For this review, take the finished solid that the model builds, in its own axes (mm). Give positions to 0.01 mm unless a question says otherwise; leave off trailing zeros. Loops run counter-clockwise (first coordinate to the right, second up) from the corner with the lowest first, then second, coordinate; pieces in that order, holes last. Notation, with made-up numbers: (41.5, 16) - (77.5, 16) arc R24 cw to (77.5, 30) - close; hole circle Ø2 at (77, -2). An arc over 180 degrees is marked (long way). Answer in a Markdown table with one row per item.
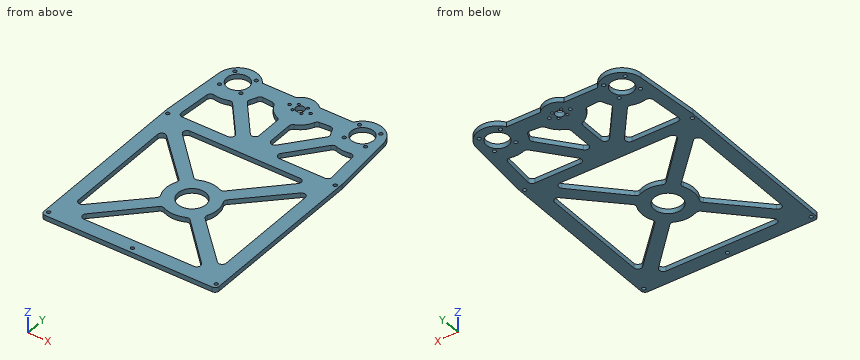
```python
from build123d import *

# Parameters (mm, degrees)
F0_R     = 2.25
F0_R_2   = 17.5
F0_R_3   = 14
F0_R_4   = 1.75
F0_R_5   = 2
F0_R_6   = 5.475
F1_DEPTH = 6


with BuildPart() as f1:
    # F0 (on Top) → F1 (new body)
    with BuildSketch(Plane.XY):
        with BuildLine():
            ThreePointArc((-94.039087, -168.43725), (-92.574621, -171.972784), (-89.039087, -173.43725))
            Line((-89.039087, -173.43725), (120.995737, -173.43725))
            ThreePointArc((120.995737, -173.43725), (124.531271, -171.972784), (125.995737, -168.43725))
            Line((125.995737, -168.43725), (125.995737, 46.355272))
            ThreePointArc((125.995737, 46.355272), (125.98705, 46.77201), (125.961003, 47.188025))
            Line((125.961003, 47.188025), (119.17908, 128.344968))
            ThreePointArc((119.17908, 128.344968), (119.244197, 127.304932), (119.265916, 126.263086))
            ThreePointArc((119.265916, 126.263086), (94.265916, 101.263086), (69.265916, 126.263086))
            ThreePointArc((69.265916, 126.263086), (70.26509, 133.260256), (73.182747, 139.698115))
            Line((73.182747, 139.698115), (30.811448, 139.698115))
            ThreePointArc((30.811448, 139.698115), (15.995916, 146.263086), (1.180383, 139.698115))
            Line((1.180383, 139.698115), (-41.190916, 139.698115))
            ThreePointArc((-41.190916, 139.698115), (-68.259772, 150.535942), (-87.186355, 128.355636))
            Line((-87.186355, 128.355636), (-94.003995, 47.190147))
            ThreePointArc((-94.003995, 47.190147), (-94.03031, 46.772005), (-94.039087, 46.353127))
            Line((-94.039087, 46.353127), (-94.039087, -168.43725))
        make_face()
        with Locations((-89.234084, -166.810914)):
            Circle(F0_R, mode=Mode.SUBTRACT)
        with BuildLine():
            ThreePointArc((-76.734085, 6.31898), (-73.661072, 10.932734), (-68.219396, 9.875237))
            Line((-68.219396, 9.875237), (-14.42265, -43.292696))
            ThreePointArc((-14.42265, -43.292696), (-13.014402, -45.974488), (-13.412905, -48.977214))
            ThreePointArc((-13.412905, -48.977214), (-16.504084, -62.810914), (-13.412905, -76.644614))
            ThreePointArc((-13.412905, -76.644614), (-13.014402, -79.64734), (-14.42265, -82.329132))
            Line((-14.42265, -82.329132), (-68.219396, -135.497065))
            ThreePointArc((-68.219396, -135.497065), (-73.661072, -136.554562), (-76.734085, -131.940809))
            Line((-76.734085, -131.940809), (-76.734085, 6.31898))
        make_face(mode=Mode.SUBTRACT)
        with Locations((15.995916, -166.810914)):
            Circle(F0_R, mode=Mode.SUBTRACT)
        with BuildLine():
            ThreePointArc((29.829615, -92.219735), (32.832342, -91.821231), (35.514134, -93.22948))
            Line((35.514134, -93.22948), (88.682067, -147.026226))
            ThreePointArc((88.682067, -147.026226), (89.739564, -152.467901), (85.12581, -155.540915))
            Line((85.12581, -155.540915), (-53.133979, -155.540915))
            ThreePointArc((-53.133979, -155.540915), (-57.747732, -152.467901), (-56.690236, -147.026226))
            Line((-56.690236, -147.026226), (-3.522302, -93.22948))
            ThreePointArc((-3.522302, -93.22948), (-0.840511, -91.821231), (2.162216, -92.219735))
            ThreePointArc((2.162216, -92.219735), (15.995916, -95.310914), (29.829615, -92.219735))
        make_face(mode=Mode.SUBTRACT)
        with Locations((121.225916, -166.810914)):
            Circle(F0_R, mode=Mode.SUBTRACT)
        with Locations((15.995916, -62.810914)):
            Circle(F0_R_2, mode=Mode.SUBTRACT)
        with BuildLine():
            ThreePointArc((45.404736, -48.977214), (45.006233, -45.974488), (46.414481, -43.292696))
            Line((46.414481, -43.292696), (100.211227, 9.875237))
            ThreePointArc((100.211227, 9.875237), (105.652903, 10.932734), (108.725916, 6.31898))
            Line((108.725916, 6.31898), (108.725916, -131.940809))
            ThreePointArc((108.725916, -131.940809), (105.652903, -136.554562), (100.211227, -135.497065))
            Line((100.211227, -135.497065), (46.414481, -82.329132))
            ThreePointArc((46.414481, -82.329132), (45.006233, -79.64734), (45.404736, -76.644614))
            ThreePointArc((45.404736, -76.644614), (48.495915, -62.810914), (45.404736, -48.977214))
        make_face(mode=Mode.SUBTRACT)
        with Locations((-89.269087, 41.189086)):
            Circle(F0_R, mode=Mode.SUBTRACT)
        with BuildLine():
            Line((-45.802034, 94.092889), (-12.476459, 53.071819))
            ThreePointArc((-12.476459, 53.071819), (-11.842592, 47.770094), (-16.357217, 44.919086))
            Line((-16.357217, 44.919086), (-73.704343, 44.919086))
            ThreePointArc((-73.704343, 44.919086), (-77.384869, 46.534751), (-78.686797, 50.337597))
            Line((-78.686797, 50.337597), (-75.349793, 90.065353))
            ThreePointArc((-75.349793, 90.065353), (-73.332149, 93.672995), (-69.288238, 94.529009))
            ThreePointArc((-69.288238, 94.529009), (-60.245963, 93.826429), (-51.36163, 95.64988))
            ThreePointArc((-51.36163, 95.64988), (-48.334397, 95.754908), (-45.802034, 94.092889))
        make_face(mode=Mode.SUBTRACT)
        with Locations((-75.709113, 112.828057)):
            Circle(F0_R, mode=Mode.SUBTRACT)
        with Locations((-75.709113, 139.698115)):
            Circle(F0_R, mode=Mode.SUBTRACT)
        with Locations((-62.274084, 126.263086)):
            Circle(F0_R_3, mode=Mode.SUBTRACT)
        with Locations((-48.839056, 112.828057)):
            Circle(F0_R, mode=Mode.SUBTRACT)
        with Locations((-48.839056, 139.698115)):
            Circle(F0_R, mode=Mode.SUBTRACT)
        with BuildLine():
            ThreePointArc((8.495916, 65.129641), (5.16867, 60.417753), (-0.384842, 61.976909))
            Line((-0.384842, 61.976909), (-34.159762, 103.551087))
            ThreePointArc((-34.159762, 103.551087), (-35.267861, 106.37018), (-34.545016, 109.311722))
            ThreePointArc((-34.545016, 109.311722), (-32.676411, 112.838194), (-31.254124, 116.567106))
            ThreePointArc((-31.254124, 116.567106), (-29.274099, 119.223089), (-26.068293, 120.058287))
            Line((-26.068293, 120.058287), (-13.708364, 119.032535))
            ThreePointArc((-13.708364, 119.032535), (-11.159348, 118.077485), (-9.488383, 115.928653))
            ThreePointArc((-9.488383, 115.928653), (-3.541995, 106.910565), (5.418993, 100.87847))
            ThreePointArc((5.418993, 100.87847), (7.656167, 99.036587), (8.495916, 96.263086))
            Line((8.495916, 96.263086), (8.495916, 65.129641))
        make_face(mode=Mode.SUBTRACT)
        with Locations((10.399165, 120.666336)):
            Circle(F0_R_4, mode=Mode.SUBTRACT)
        with Locations((2.795916, 126.263086)):
            Circle(F0_R_5, mode=Mode.SUBTRACT)
        with Locations((10.399165, 131.859836)):
            Circle(F0_R_4, mode=Mode.SUBTRACT)
        with BuildLine():
            ThreePointArc((2.162216, -33.402094), (-0.840511, -33.800597), (-3.522302, -32.392349))
            Line((-3.522302, -32.392349), (-56.690236, 21.404398))
            ThreePointArc((-56.690236, 21.404398), (-57.747732, 26.846073), (-53.133979, 29.919086))
            Line((-53.133979, 29.919086), (85.12581, 29.919086))
            ThreePointArc((85.12581, 29.919086), (89.739564, 26.846073), (88.682067, 21.404398))
            Line((88.682067, 21.404398), (35.514134, -32.392349))
            ThreePointArc((35.514134, -32.392349), (32.832342, -33.800597), (29.829615, -33.402094))
            ThreePointArc((29.829615, -33.402094), (15.995916, -30.310915), (2.162216, -33.402094))
        make_face(mode=Mode.SUBTRACT)
        with Locations((121.225916, 41.189086)):
            Circle(F0_R, mode=Mode.SUBTRACT)
        with BuildLine():
            Line((23.495916, 65.129641), (23.495916, 96.263086))
            ThreePointArc((23.495916, 96.263086), (24.335664, 99.036587), (26.572839, 100.87847))
            ThreePointArc((26.572839, 100.87847), (35.533826, 106.910565), (41.480215, 115.928653))
            ThreePointArc((41.480215, 115.928653), (43.151179, 118.077485), (45.700195, 119.032535))
            Line((45.700195, 119.032535), (58.060124, 120.058287))
            ThreePointArc((58.060124, 120.058287), (61.26593, 119.223089), (63.245955, 116.567106))
            ThreePointArc((63.245955, 116.567106), (64.668242, 112.838194), (66.536847, 109.311722))
            ThreePointArc((66.536847, 109.311722), (67.259692, 106.37018), (66.151593, 103.551087))
            Line((66.151593, 103.551087), (32.376673, 61.976909))
            ThreePointArc((32.376673, 61.976909), (26.823161, 60.417753), (23.495916, 65.129641))
        make_face(mode=Mode.SUBTRACT)
        with Locations((21.592666, 120.666336)):
            Circle(F0_R_4, mode=Mode.SUBTRACT)
        with Locations((15.995916, 126.263086)):
            Circle(F0_R_6, mode=Mode.SUBTRACT)
        with BuildLine():
            ThreePointArc((27.195916, 126.263086), (29.195916, 128.263086), (31.195916, 126.263086))
            ThreePointArc((31.195916, 126.263086), (29.195916, 124.263086), (27.195916, 126.263086))
        make_face(mode=Mode.SUBTRACT)
        with Locations((21.592666, 131.859836)):
            Circle(F0_R_4, mode=Mode.SUBTRACT)
        with BuildLine():
            ThreePointArc((48.349048, 44.919086), (43.834424, 47.770094), (44.46829, 53.071819))
            Line((44.46829, 53.071819), (77.793865, 94.092889))
            ThreePointArc((77.793865, 94.092889), (80.326229, 95.754908), (83.353462, 95.64988))
            ThreePointArc((83.353462, 95.64988), (92.237795, 93.826429), (101.280069, 94.529009))
            ThreePointArc((101.280069, 94.529009), (105.32398, 93.672995), (107.341624, 90.065353))
            Line((107.341624, 90.065353), (110.678628, 50.337597))
            ThreePointArc((110.678628, 50.337597), (109.3767, 46.534751), (105.696174, 44.919086))
            Line((105.696174, 44.919086), (48.349048, 44.919086))
        make_face(mode=Mode.SUBTRACT)
        with BuildLine():
            ThreePointArc((119.265916, 126.263086), (119.244197, 127.304932), (119.17908, 128.344968))
            ThreePointArc((119.17908, 128.344968), (100.256801, 150.53466), (73.182747, 139.698115))
            ThreePointArc((73.182747, 139.698115), (70.26509, 133.260256), (69.265916, 126.263086))
            ThreePointArc((69.265916, 126.263086), (94.265916, 101.263086), (119.265916, 126.263086))
        make_face()
        with Locations((80.830887, 112.828057)):
            Circle(F0_R, mode=Mode.SUBTRACT)
        with Locations((94.265916, 126.263086)):
            Circle(F0_R_3, mode=Mode.SUBTRACT)
        with Locations((80.830887, 139.698115)):
            Circle(F0_R, mode=Mode.SUBTRACT)
        with Locations((107.700944, 112.828057)):
            Circle(F0_R, mode=Mode.SUBTRACT)
        with Locations((107.700944, 139.698115)):
            Circle(F0_R, mode=Mode.SUBTRACT)
    extrude(amount=F1_DEPTH)


solid = f1.part
```
1. We need section A-A, the plane x = -21.5. Give the boundary of the cut face in (y, z), and give its area (3 significant figures).
Values:
| item | result |
|---|---|
| outline | (-173.44, 0) - (-155.54, 0) - (-155.54, 6) - (-173.44, 6) - close; (-111.42, 0) - (-89.32, 0) - (-89.32, 6) - (-111.42, 6) - close; (-36.3, 0) - (-14.2, 0) - (-14.2, 6) - (-36.3, 6) - close; (29.92, 0) - (44.92, 0) - (44.92, 6) - (29.92, 6) - close; (64.18, 0) - (87.97, 0) - (87.97, 6) - (64.18, 6) - close; (119.68, 0) - (139.7, 0) - (139.7, 6) - (119.68, 6) - close |
| area | 725 mm^2 |
2. We need section C-C, the plane z = 5.05. Count the separate pieces of the cut face and the enclosed holes in it, and give its area (3 significant figures).
Values:
| item | result |
|---|---|
| separate pieces | 1 |
| enclosed holes | 31 |
| area | 33,700 mm^2 |
3. We need section B-B, the plane y = -142. Give the boundary of the cut face in (x, z).
Values:
| item | result |
|---|---|
| outline | (-94.04, 0) - (-51.72, 0) - (-51.72, 6) - (-94.04, 6) - close; (83.71, 0) - (126, 0) - (126, 6) - (83.71, 6) - close |
4. Wall thickness on line 1 (X direction, y = -59, z = 3.35); line 2 (Y direction, x = 99, z = 3); line 3 (X direction, y = -98, z = 4.6): over which ranges is each line inside the solid? List them lowest first. Write a range as [from, to].
Values:
| item | result |
|---|---|
| line 1 | x = [-94.04, -76.73], [-16.28, -1.08], [33.08, 48.27], [108.73, 126] |
| line 2 | y = [-173.44, -134.3], [8.68, 44.92], [94.11, 113.09], [139.44, 150.81] |
| line 3 | x = [-94.04, -76.73], [-30.28, -8.24], [40.23, 62.27], [108.73, 126] |
5. Clearance check with flat-ended pins moving along their axes: pin 1 (2 mm diameter, centred on x = 21.59, y = 131.86, fed in from -Z); pin 2 (2 mm diameter, centred on x = -40.5, z = 3, fed in from +Y); pin 3 (1.5 mm diameter, centred on x = 20, z = 5, fed in from +Y). State where each tip first meets the part, or that it passes through.
Values:
| item | result |
|---|---|
| pin 1 | passes through |
| pin 2 | stops at y = 140.17 |
| pin 3 | stops at y = 146 |
